from build123d import *

# Parameters (mm, degrees)
SKETCH1_W           = 57
SKETCH1_H           = 57
BOSS_EXTRUDE1_DEPTH = 12
FILLET1_R           = 5
SKETCH2_R           = 2.5
SKETCH2_R_2         = 1.7
CUT_EXTRUDE1_DEPTH  = 43.053537307
CIRPATTERN2_COUNT   = 4
SKETCH3_R           = 27
CUT_EXTRUDE2_DEPTH  = 1
SKETCH4_R           = 25.05
CUT_EXTRUDE3_DEPTH  = 2
CHAMFER1_SIZE       = 1
SKETCH5_R           = 24.05
CUT_EXTRUDE4_DEPTH  = 8
SKETCH6_R           = 23.5
CUT_EXTRUDE5_DEPTH  = 2
BOSS_EXTRUDE2_DEPTH = 1
CIRPATTERN3_COUNT   = 4
CUT_EXTRUDE8_START  = -3
SKETCH9_R           = 3
SKETCH9_R_2         = 1.7
CUT_EXTRUDE8_DEPTH  = 3
CIRPATTERN6_COUNT   = 4


with BuildPart() as part:
    # Sketch1 → Boss-Extrude1 (new body)
    with BuildSketch(Plane(origin=(0, 0, 0), x_dir=(1, 0, 0), z_dir=(0, 1, 0))):
        Rectangle(SKETCH1_W, SKETCH1_H)
    extrude(amount=BOSS_EXTRUDE1_DEPTH)

    # Fillet1
    fillet1_edges = [part.edges().sort_by_distance(p)[0] for p in [
        (-28.5, 6, -28.5),
        (28.5, 6, -28.5),
        (28.5, 6, 28.5),
        (-28.5, 6, 28.5),
    ]]
    fillet(fillet1_edges, radius=FILLET1_R)

    # Sketch2 → Cut-Extrude1 (cut, through all)
    with BuildSketch(Plane(origin=(0, 12, 0), x_dir=(1, 0, 0), z_dir=(0, 1, 0))):
        with Locations(Location((-23.5, 23.5, 0), (0, 0, 270))):
            Circle(SKETCH2_R)
        with Locations(Location((-25, 15.5, 0), (0, 0, 270))):
            Circle(SKETCH2_R_2)
    cut_extrude1 = extrude(amount=-CUT_EXTRUDE1_DEPTH, mode=Mode.SUBTRACT)

    # CirPattern2: Cut-Extrude1 ×4 about axis
    cirpattern2_axis = Axis((0.215204442, 0, 0.188240663), (0, 1, 0))
    for i in range(1, CIRPATTERN2_COUNT):
        add(cut_extrude1.rotate(cirpattern2_axis, i * 360 / CIRPATTERN2_COUNT), mode=Mode.SUBTRACT)

    # Sketch3 → Cut-Extrude2 (cut)
    with BuildSketch(Plane(origin=(0, 12, 0), x_dir=(1, 0, 0), z_dir=(0, 1, 0))):
        with Locations(Location((0, 0, 0), (0, 0, 270))):
            Circle(SKETCH3_R)
    extrude(amount=-CUT_EXTRUDE2_DEPTH, mode=Mode.SUBTRACT)

    # Sketch4 → Cut-Extrude3 (cut)
    with BuildSketch(Plane(origin=(0, 11, 0), x_dir=(1, 0, 0), z_dir=(0, 1, 0))):
        with Locations(Location((0, 0, 0), (0, 0, 270))):
            Circle(SKETCH4_R)
    extrude(amount=-CUT_EXTRUDE3_DEPTH, mode=Mode.SUBTRACT)

    # Chamfer1
    chamfer1_edges = [part.edges().sort_by_distance(p)[0] for p in [
        (0, 9, -25.05),
    ]]
    chamfer(chamfer1_edges, length=CHAMFER1_SIZE)

    # Sketch5 → Cut-Extrude4 (cut)
    with BuildSketch(Plane(origin=(0, 9, 0), x_dir=(1, 0, 0), z_dir=(0, 1, 0))):
        with Locations(Location((0, 0, 0), (0, 0, 270))):
            Circle(SKETCH5_R)
    extrude(amount=-CUT_EXTRUDE4_DEPTH, mode=Mode.SUBTRACT)

    # Sketch6 → Cut-Extrude5 (cut)
    with BuildSketch(Plane(origin=(0, 1, 0), x_dir=(1, 0, 0), z_dir=(0, 1, 0))):
        with Locations(Location((0, 0, 0), (0, 0, 270))):
            Circle(SKETCH6_R)
    extrude(amount=-CUT_EXTRUDE5_DEPTH, mode=Mode.SUBTRACT)

    # Sketch7 → Boss-Extrude2 (add)
    with BuildSketch(Plane(origin=(0, 12, 0), x_dir=(1, 0, 0), z_dir=(0, 1, 0))):
        Polygon((27.5, 0), (27.5, -11), (28.5, -11.996579712), (28.5, 0), align=None)
        Polygon((27.5, 11), (27.5, 0), (28.5, 0), (28.5, 11.996579712), align=None)
    boss_extrude2 = extrude(amount=BOSS_EXTRUDE2_DEPTH)

    # CirPattern3: Boss-Extrude2 ×4 about axis
    cirpattern3_axis = Axis((0, 0, 0), (0, 1, 0))
    for i in range(1, CIRPATTERN3_COUNT):
        add(boss_extrude2.rotate(cirpattern3_axis, i * 360 / CIRPATTERN3_COUNT))

    # Sketch9 → Cut-Extrude8 (cut)
    # profile 1 of 3: a face of its own
    with BuildSketch(Plane.XZ.offset(CUT_EXTRUDE8_START)):
        with Locations((-15.473036222, 25.403445105)):
            Circle(SKETCH9_R)
        with Locations((-15.473036222, 25.403445105)):
            Circle(SKETCH9_R_2, mode=Mode.SUBTRACT)
    # profile 2 of 3: a face of its own
    with BuildSketch(Plane.XZ.offset(CUT_EXTRUDE8_START)):
        with BuildLine():
            ThreePointArc((-18.473036222, 25.403445105), (-15.473036222, 28.403445105), (-12.473036222, 25.403445105))
            Line((-12.473036222, 25.403445105), (-12.473036222, 28.424359567))
            Line((-12.473036222, 28.424359567), (-12.473036222, 28.5))
            Line((-12.473036222, 28.5), (-18.473036222, 28.5))
            Line((-18.473036222, 28.5), (-18.473036222, 25.403445105))
        make_face()
    # profile 3 of 3: a face of its own
    with BuildSketch(Plane.XZ.offset(CUT_EXTRUDE8_START)):
        with Locations((-15.473036222, 25.403445105)):
            Circle(SKETCH9_R_2)
    cut_extrude8 = extrude(amount=CUT_EXTRUDE8_DEPTH, mode=Mode.SUBTRACT)

    # CirPattern6: Cut-Extrude8 ×4 about axis
    cirpattern6_axis = Axis((0, 0, 0), (0, 1, 0))
    for i in range(1, CIRPATTERN6_COUNT):
        add(cut_extrude8.rotate(cirpattern6_axis, i * 360 / CIRPATTERN6_COUNT), mode=Mode.SUBTRACT)


solid = part.part
Here's how the part is built. I have some questions about the finished solid (model axes, mm). A direction names the side the tool comes from. Coordinates: 2 decimals unless noted, no trailing zeros. Order: outer loops, then holes, each group sorted by start corner. A loop starts at its lowest first (then second) coordinate and runs counter-clockwise, first axis right, second up. Notation, with made-up numbers: (85.25, -37) - (138.25, -37) arc R15 cw to (138.25, -22) - close; hole circle Ø8 at (56.25, 84). An arc over 180 degrees is marked (long way). Use CSV: the item, a comma, the result in double quotes. Start each with the question number.
1. For faces 4 (the face through (12.473, 2, -27)), 5 (the face through (-27, 2, -12.473)), 6 (the face through (-18.473, 2, 27)), 7 (the face through (26, 3, 14)), 8 (the face through (7.5, 10.5, 23.9)), which set-ups out of +Z, -Z, +X, -X, +Y, -Y let a thin tool reach every point of the face, with its end or its side?
2. If we mould it in two halves opening along X, with no side actions, what happens to faces 1 (the face through (0, 0, -26)), 2 (the face through (-27.07, 6.08, 27)), 3 (the face through (-8, 11, 24))? For each: +X half, -X half, draft (parallel to the pull), parting line (faces both ways), or undercut.
3. Suppose I cut it at A-A on x = 0. List the corners of the cut face in (y, z) for me, then the cut area to 3 significant figures.
4. Suppose I cut it at C-C on y = 5.25. Give the number of separate pieces and of enclosed holes in the cut face, then the cut area to 3 significant figures.
5. I'm going to push flat-ended pins straight in: pin 1 (1.8 mm diameter, centred on x = -27, z = -14.5, fed in from -Y); pin 2 (1.5 mm diameter, centred on y = 1.5, z = -27.5, fed in from -X); pin 3 (1.5 mm diameter, centred on y = 2, z = 27, fed in from +X). Where does each tip first touch, or does it pass through?
6. Suppose I cut it at B-B on z = 0. List the corners of the cut face in (x, y) for me, then the cut area to 3 significant figures.
7. Please list where these lines run through material, in increasing order: line 1 (X direction, y = 2.5, z = 0.5); line 2 (X direction, y = 5, z = -24.5); line 3 (X direction, y = 10.75, z = -15). Write a range as from..to.
Output:
1,face 4,"-Z, -Y"
1,face 5,"-X, -Y"
1,face 6,"+Z, -Y"
1,face 7,"+X, -Y"
1,face 8,"+Y"
2,face 1,"draft"
2,face 2,"-X half"
2,face 3,"undercut"
3,outline,"(0, -28.5) - (13, -28.5) - (13, -27.5) - (12, -27.5) - (12, -27) - (11, -27) - (11, -25.05) - (10, -25.05) - (9, -24.05) - (1, -24.05) - (1, -23.5) - (0, -23.5) - close; (0, 23.5) - (1, 23.5) - (1, 24.05) - (9, 24.05) - (10, 25.05) - (11, 25.05) - (11, 27) - (12, 27) - (12, 27.5) - (13, 27.5) - (13, 28.5) - (0, 28.5) - close"
3,area,"101 mm2"
4,separate pieces,"1"
4,enclosed holes,"9"
4,area,"1,300 mm2"
5,pin 1,"stops at y = 3"
5,pin 2,"stops at x = -27.3"
5,pin 3,"stops at x = 27.68"
6,outline,"(-28.5, 0) - (-23.5, 0) - (-23.5, 1) - (-24.05, 1) - (-24.05, 9) - (-25.05, 10) - (-25.05, 11) - (-27, 11) - (-27, 12) - (-27.5, 12) - (-27.5, 13) - (-28.5, 13) - close; (23.5, 0) - (28.5, 0) - (28.5, 13) - (27.5, 13) - (27.5, 12) - (27, 12) - (27, 11) - (25.05, 11) - (25.05, 10) - (24.05, 9) - (24.05, 1) - (23.5, 1) - close"
6,area,"101 mm2"
7,line 1,"x = -28.5..-24.04, 24.04..28.5"
7,line 2,"x = -28.4..-25.79, -21.21..14.29, 17.52..21.6, 26.21..28.4"
7,line 3,"x = -28.5..-26.62, -23.38..-20.06, 20.06..28.5"
